Check sheet for the modelled part. Datum: model origin and axes. Units: mm. Face numbers are marked on the shaded views. Give positions to 0.01 mm unless a question says otherwise; leave off trailing zeros. Loops run counter-clockwise (first coordinate to the right, second up) from the corner with the lowest first, then second, coordinate; pieces in that order, holes last. Notation, with made-up numbers: M 46.25,13.5 L 99.25,13.5 A33 cw 99.25,42.5 Z; hole C 22.25,35 d9. An arc over 180 degrees is marked long. Use one line per item in the form item = value.
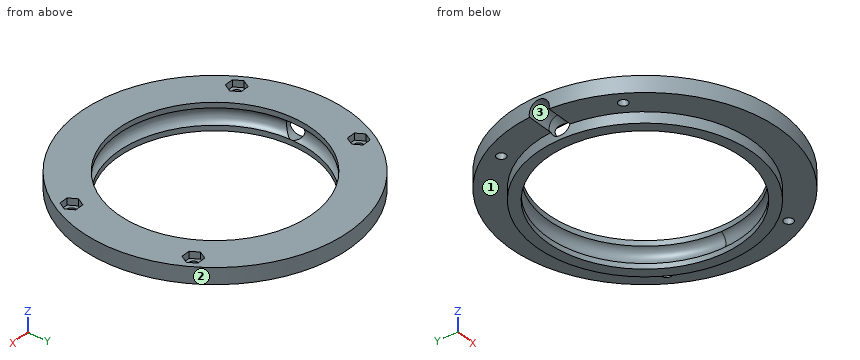
from build123d import *

# Parameters (mm, degrees)
SKETCH002_R     = 1.7
POCKET_DEPTH    = 10.001
POCKET001_DEPTH = 2.5


with BuildPart() as part:
    # Sketch → Revolution (revolve)
    with BuildSketch(Plane.XZ):
        with BuildLine():
            ThreePointArc((36, 1.960263), (38.2, 5), (36, 8.039737))
            Line((36, 8.039737), (36, 10))
            Line((36, 10), (50, 10))
            Line((50, 10), (50, 4))
            Line((50, 4), (40, 4))
            Line((40, 4), (40, 0))
            Line((40, 0), (36, 0))
            Line((36, 0), (36, 1.960263))
        make_face()
    revolve(axis=Axis((0, 0, 0), (0, 0, 1)))

    # Sketch001 (on DatumPlane) → Groove (revolve, cut)
    with BuildSketch(Plane.XY.offset(5)):
        Polygon((-35.5, 0), (-35.5, 3), (-40.5, 3.7), (-51.5, 3.7), (-51.5, 0), align=None)
    revolve(axis=Axis((0, 0, 5), (1, 0, 0)), mode=Mode.SUBTRACT)

    # Sketch002 (on Face6 of Groove) → Pocket (cut, through all)
    with BuildSketch(Plane(origin=(0, 0, 10), x_dir=(-1, 0, 0), z_dir=(0, 0, 1))):
        with Locations((39, -22.5)):
            Circle(SKETCH002_R)
        with Locations((39, 22.5)):
            Circle(SKETCH002_R)
        with Locations((-39, 22.5)):
            Circle(SKETCH002_R)
        with Locations((-39, -22.5)):
            Circle(SKETCH002_R)
    extrude(amount=-POCKET_DEPTH, mode=Mode.SUBTRACT)

    # Sketch003 (on Face6 of Pocket) → Pocket001 (cut)
    with BuildSketch(Plane(origin=(0, 0, 10), x_dir=(-1, 0, 0), z_dir=(0, 0, 1))):
        Polygon((37.325, 25.401185), (35.65, 22.5), (37.325, 19.598815), (40.675, 19.598815), (42.35, 22.5), (40.675, 25.401185), align=None)
        Polygon((-37.325, 25.401185), (-40.675, 25.401185), (-42.35, 22.5), (-40.675, 19.598815), (-37.325, 19.598815), (-35.65, 22.5), align=None)
        Polygon((-37.325, -19.598815), (-40.675, -19.598815), (-42.35, -22.5), (-40.675, -25.401185), (-37.325, -25.401185), (-35.65, -22.5), align=None)
        Polygon((40.675, -19.598815), (37.325, -19.598815), (35.65, -22.5), (37.325, -25.401185), (40.675, -25.401185), (42.35, -22.5), align=None)
    extrude(amount=-POCKET001_DEPTH, mode=Mode.SUBTRACT)


solid = part.part
1) Section check A-A (x = 0). Record the cut outline in (y, z), then the cut area to 3 significant figures.
Evaluation:
outline = M -50,4 L -40,4 L -40,0 L -36,0 L -36,1.96 A3.2 cw -36,8.04 L -36,10 L -50,10 Z; M 36,0 L 40,0 L 40,4 L 50,4 L 50,10 L 36,10 L 36,8.04 A3.2 cw 36,1.96 Z
area = 180 mm^2
2) Release check for a two-part mould opening along Y. For the marked faces 1, 2 and 3 record: pulls with the +Y half, pulls with the -Y half, needs draft (parallel to the pull), parting line crosses it, or undercut.
Evaluation:
face_1 = needs draft
face_2 = parting line crosses it
face_3 = undercut
3) Depth check by flat-ended pin: pin 1 Ø5 at (y, z) = (-17, 3) entering from -X; pin 2 Ø1.2 at (x, z) = (39, 8.5) entering from -Y; pin 3 Ø4 at (x, z) = (-8.5, 4.5) entering from +Y; pin 4 Ø3 at (x, y) = (-39, -22.5) entering from +Z. Enter the tip coordinate at first touch or a pass-through.
Evaluation:
pin_1 = -47.79
pin_2 = -32.02
pin_3 = 49.58
pin_4 = through
4) Scan lines: line 1 (X direction, y = 22.5, z = 5.95); line 2 (X direction, y = 0, z = 1.05); line 3 (X direction, y = 22.5, z = 5). Record each from-to range of solid material in increasing order.
Evaluation:
line_1 = -44.65 to -40.7, -37.3 to -30.69, 30.69 to 37.3, 40.7 to 44.65
line_2 = -40 to -36, 36 to 40
line_3 = -44.65 to -40.7, -37.3 to -30.87, 30.87 to 37.3, 40.7 to 44.65
